For this review, use the dimensioned drawing (mm, ordinates from the lowest corner) and the shaded views. Give positions to 0.01 mm unless a question says otherwise; leave off trailing zeros. Loops run counter-clockwise (first coordinate to the right, second up) from the corner with the lowest first, then second, coordinate; pieces in that order, holes last. Notation, with made-up numbers: M 46.25,63 L 59.25,63 A21 ccw 59.25,101 Z; hole C -13.75,-9.5 d4. An arc over 180 degrees is marked long. Use CSV: the item, a comma, the result in double quotes.
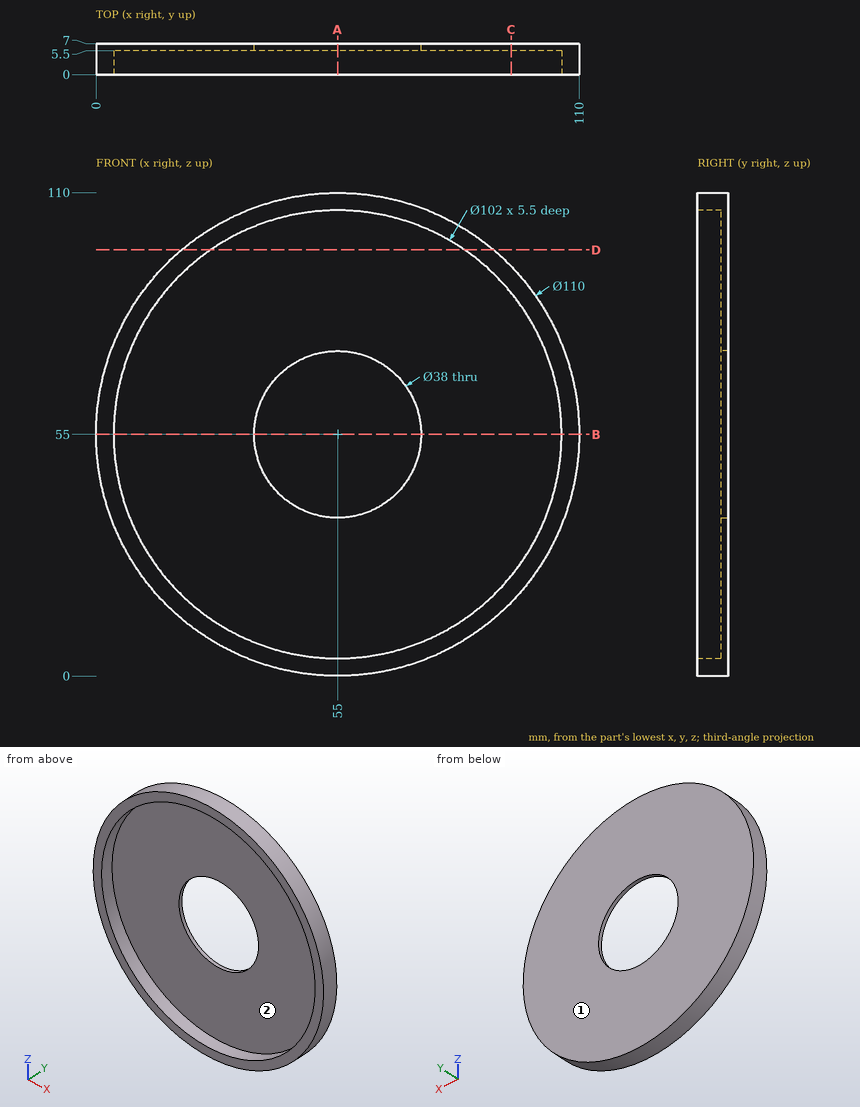
(1) The part is to be moulded in two halves that separate along X. For the marked faces 1 and 2, say which applies: released by +X, released by -X, zero draft, split by the parting line, or undercut.
A:
face 1,"zero draft"
face 2,"undercut"
(2) Wall thickness on line 1 along X through (y, z) = (5.9, 55); line 2 along X through (y, z) = (0.5, 53.5); line 3 along Y through (x, z) = (50, 31): over which ranges is each line inside the solid? List them lowest first. Write a range as [from, to].
A:
line 1,"[0, 36], [74, 110]"
line 2,"[0.02, 4.02], [105.98, 109.98]"
line 3,"[5.5, 7]"
(3) We need section B-B on z = 55. State the section outline as (x, y) points.
A:
outline,"M 0,0 L 4,0 L 4,5.5 L 36,5.5 L 36,7 L 0,7 Z; M 74,5.5 L 106,5.5 L 106,0 L 110,0 L 110,7 L 74,7 Z"
(4) We need section A-A on x = 55. State the section outline as (y, z) points.
A:
outline,"M 0,0 L 7,0 L 7,36 L 5.5,36 L 5.5,4 L 0,4 Z; M 0,106 L 5.5,106 L 5.5,74 L 7,74 L 7,110 L 0,110 Z"
(5) Clearance check with flat-ended pins moving along their axes: P1, Ø3, axis at y = 6, z = 19, coming from the -X side; P2, Ø1, axis at x = 46, y = 1, coming from the +Z side; P3, Ø3, axis at x = 53, z = 76, coming from the -Y side. State where each tip first meets the part, or that it passes through.
A:
P1,"x = 12.17"
P2,"z = 109.34"
P3,"y = 5.5"
(6) We need section C-C on x = 94.5. State the section outline as (y, z) points, then the cut area to 3 significant figures.
A:
outline,"M 0,16.73 L 7,16.73 L 7,93.27 L 0,93.27 L 0,87.26 L 5.5,87.26 L 5.5,22.74 L 0,22.74 Z"
area,"181 mm²"
(7) We need section D-D on z = 97. State the section outline as (x, y) points, then the cut area to 3 significant figures.
A:
outline,"M 19.49,0 L 26.07,0 L 26.07,5.5 L 83.93,5.5 L 83.93,0 L 90.51,0 L 90.51,7 L 19.49,7 Z"
area,"179 mm²"
